Source: CAD feature listing. Evaluate the final solid. Frame: model axes, mm. A direction names the side the tool comes from. Give positions to 0.01 mm unless a question says otherwise; leave off trailing zeros. Order: outer loops, then holes, each group sorted by start corner. A loop starts at its lowest first (then second) coordinate and runs counter-clockwise, first axis right, second up.
```python
from build123d import *

# Parameters (mm, degrees)
SKETCH1_R           = 52.5
BOSS_EXTRUDE1_DEPTH = 6
SKETCH2_R           = 5
CUT_EXTRUDE1_DEPTH  = 75.488254108
SKETCH3_R           = 7.120379286
CUT_EXTRUDE2_DEPTH  = 4.924026
CIRPATTERN1_START   = 1.075974424
CIRPATTERN1_DEPTH   = 4.924025576


# Read off the part's stored shape, not the designer's step: CirPattern1
with BuildPart() as part:
    # Sketch1 → Boss-Extrude1 (new body)
    with BuildSketch(Plane(origin=(0, 0, 0), x_dir=(1, 0, 0), z_dir=(0, 1, 0))):
        with Locations(Location((0, 0, 0), (0, 0, 270))):
            Circle(SKETCH1_R)
    extrude(amount=BOSS_EXTRUDE1_DEPTH)

    # Sketch2 → Cut-Extrude1 (cut, through all)
    with BuildSketch(Plane(origin=(0, 0, 0), x_dir=(1, 0, 0), z_dir=(0, 1, 0))):
        with Locations(Location((0, 0, 0), (0, 0, 270))):
            Circle(SKETCH2_R)
    extrude(amount=CUT_EXTRUDE1_DEPTH, mode=Mode.SUBTRACT)

    # Sketch3 → Cut-Extrude2 (cut)
    with BuildSketch(Plane(origin=(0, 6, 0), x_dir=(1, 0, 0), z_dir=(0, 1, 0))):
        with Locations((-7.922010369, 0)):
            Circle(SKETCH3_R)
    extrude(amount=-CUT_EXTRUDE2_DEPTH, mode=Mode.SUBTRACT)

    # CirPattern1 outline → CirPattern1 (cut)
    with BuildSketch(Plane(origin=(0, 0, 0), x_dir=(1, 0, 0), z_dir=(0, 1, 0)).offset(CIRPATTERN1_START)):
        with BuildLine():
            ThreePointArc((-2.338954722, -4.41919572), (-4.441940414, -6.211997608), (-7.069113695, -7.069113695))
            ThreePointArc((-7.069113695, -7.069113695), (0, -15.042389655), (7.069113695, -7.069113695))
            ThreePointArc((7.069113695, -7.069113695), (15.042389655, 0), (7.069113695, 7.069113695))
            ThreePointArc((7.069113695, 7.069113695), (0, 15.042389655), (-7.069113695, 7.069113695))
            ThreePointArc((-7.069113695, 7.069113695), (-4.441940414, 6.211997608), (-2.338954722, 4.41919572))
            ThreePointArc((-2.338954722, 4.41919572), (5, 0), (-2.338954722, -4.41919572))
        make_face()
    extrude(amount=CIRPATTERN1_DEPTH, mode=Mode.SUBTRACT)


solid = part.part
```
1) Section query C-C, the plane y = 2.25. Return the cut outline in (x, z), and give its area (3 significant figures).
Report:
outline: circle Ø105 at (0, 0); hole (-7.07, -7.07) arc R7.12 ccw (long way) to (7.07, -7.07) arc R7.12 ccw (long way) to (7.07, 7.07) arc R7.12 ccw (long way) to (-7.07, 7.07) arc R7.12 ccw (long way) to start
area: 8,090 mm2
2) Section query D-D, the plane z = 46.5. Return the cut outline in (x, y), and give its area (3 significant figures).
Report:
outline: (-24.37, 0) - (24.37, 0) - (24.37, 6) - (-24.37, 6) - close
area: 292 mm2
3) Material intervals for L1, parallel to X at y = 3.45, z = 0; L2, parallel to X at y = 0.65, z = 0; L3, parallel to Z at x = -13.5, y = 3.8, sorted ascending.
Report:
L1: x = -52.5 to -15.04, 15.04 to 52.5
L2: x = -52.5 to -5, 5 to 52.5
L3: z = -50.73 to -4.43, 4.43 to 50.73
4) Draft query along Z for faces 1 (the cylindrical face through (1.5, 0.53, 4.77)), 2 (the cylindrical face through (15.77, 2.958, 50.076)), 3 (the flat face through (-11, 6, 11)). Return one class per face: +Z half, -Z half, draft (parallel to the pull), parting line (faces both ways), or undercut.
Report:
face 1: undercut
face 2: parting line
face 3: draft
5) Section query A-A, the plane z = 0. Return the cut outline in (x, y), and give its area (3 significant figures).
Report:
outline: (-52.5, 0) - (-5, 0) - (-5, 1.08) - (-15.04, 1.08) - (-15.04, 6) - (-52.5, 6) - close; (5, 0) - (52.5, 0) - (52.5, 6) - (15.04, 6) - (15.04, 1.08) - (5, 1.08) - close
area: 471 mm2
6) Section query B-B, the plane x = 0. Return the cut outline in (y, z).
Report:
outline: (0, -52.5) - (6, -52.5) - (6, -15.04) - (1.08, -15.04) - (1.08, -5) - (0, -5) - close; (0, 5) - (1.08, 5) - (1.08, 15.04) - (6, 15.04) - (6, 52.5) - (0, 52.5) - close
7) Reachability of faces 4 (the flat face through (-11, 0, -1)), 5 (the cylindrical face through (15.04, 3.5, 0.17)) from +Z, -Z, +X, -X, +Y, -Y: full face, straight path, thin tool, end or side. Return the list, or none.
Report:
face 4: +Z, -Z, +X, -X, -Y
face 5: +Y
8) Pin query (flat end, axial travel): pin 1 (13 mm diameter, centred on x = 0, z = 0, fed in from +Y); pin 2 (1 mm diameter, centred on y = 5, z = 22.5, fed in from +X); pin 3 (2 mm diameter, centred on x = 14, y = 3.5, fed in from +Z) (3 decimals). Return the tip coordinate at first contact, or that it passes through.
Report:
pin 1: stops at y = 1.08
pin 2: stops at x = 47.67
pin 3: stops at z = 50.865
